```python
from build123d import *

# Parameters (mm, degrees)
F1_DEPTH = 5.2
F3_DEPTH = 25.4


with BuildPart() as f1:
    # F0 (on Front) → F1 (new body)
    with BuildSketch(Plane.XZ):
        Polygon((1.5, 0), (0, 0), (0, -12), (12, -12), (12, -10.8), (1.5, -10.8), align=None)
    extrude(amount=-F1_DEPTH)

    # F2 (on face) → F3 (cut)
    with BuildSketch(Plane.YZ.offset(1.5)):
        with BuildLine():
            Line((1.1, -2.9), (1.1, -7.9))
            ThreePointArc((1.1, -7.9), (2.575413, -9.400208), (4.1, -7.95))
            Line((4.1, -7.95), (4.1, -2.9))
            ThreePointArc((4.1, -2.9), (2.6, -1.4), (1.1, -2.9))
        make_face()
    extrude(amount=-F3_DEPTH, mode=Mode.SUBTRACT)


solid = f1.part
```
Check sheet for the modelled part. Datum: model origin and axes. Units: mm. A direction names the side the tool comes from. Round coordinates to 2 decimals unless told otherwise and drop trailing zeros. Order: outer loops, then holes, each group sorted by start corner. A loop starts at its lowest first (then second) coordinate and runs counter-clockwise, first axis right, second up. Notation, with made-up numbers: (16, 81) -> (59, 81) arc R26 ccw to (59, 114) -> close; hole circle Ø4 at (-30, 63). An arc over 180 degrees is marked (long way). One line per item, written item: value. Start each with the question number.
Q1. Cross-section at C-C (y = 4.7). Record the boundary of the cut face in (x, z).
Q2. Cross-section at D-D (y = 3.35). Record the boundary of the cut face in (x, z).
Q3. Mould release check, pull along Z, two halves, no side actions. Record for faces 1 (the face through (3, 5.2, -11)), 2 (the face through (1, 1.1, -5)), 3 (the face through (1, 3, 0)): pulls with the +Z half, pulls with the -Z half, needs draft (parallel to the pull), parting line crosses it, or undercut.
Q4. Cross-section at A-A (z = -3.5). Record the boundary of the cut face in (x, y).
Q5. Gauge pin test, flat ends, axial feed: pin 1 Ø1.5 at (x, z) = (4, -4) entering from +Y; pin 2 Ø1.2 at (x, z) = (1, -5.5) entering from -Y. Record the tip position at first contact, or that the pin passes through.
Q6. Cross-section at B-B (y = 2.6). Record the boundary of the cut face in (x, z), and give its area (3 significant figures).
Q7. Thickness scan on line 1 (Y direction, x = 0.5, z = -4); line 2 (Z direction, x = 11, y = 4.55); line 3 (X direction, y = 5, z = -9.5). Record the ranges inside material, lowest first.
Q8. Set-up check for faces 4 (the face through (7, 3, -10.8)), 5 (the face through (0.76, 2.54, -9.4)), 6 (the face through (3, 0, -11)): record each of +Z, -Z, +X, -X, +Y, -Y from which the full face is reachable in a straight line by a thin tool's end or side.
Completed:
1. outline: (0, -12) -> (12, -12) -> (12, -10.8) -> (1.5, -10.8) -> (1.5, 0) -> (0, 0) -> close
2. outline: (0, -12) -> (12, -12) -> (12, -10.8) -> (1.5, -10.8) -> (1.5, -9.2) -> (0, -9.2) -> close; (0, -1.6) -> (1.5, -1.6) -> (1.5, 0) -> (0, 0) -> close
3. face 1: needs draft
3. face 2: undercut
3. face 3: pulls with the +Z half
4. outline: (0, 0) -> (1.5, 0) -> (1.5, 1.1) -> (0, 1.1) -> close; (0, 4.1) -> (1.5, 4.1) -> (1.5, 5.2) -> (0, 5.2) -> close
5. pin 1: passes through
5. pin 2: stops at y = 0
6. outline: (0, -12) -> (12, -12) -> (12, -10.8) -> (1.5, -10.8) -> (1.5, -9.4) -> (0, -9.4) -> close; (0, -1.4) -> (1.5, -1.4) -> (1.5, 0) -> (0, 0) -> close
6. area: 18.6 mm²
7. line 1: y = 0 to 1.1, 4.1 to 5.2
7. line 2: z = -12 to -10.8
7. line 3: x = 0 to 1.5
8. face 4: +Z, +X, +Y, -Y
8. face 5: +X, -X
8. face 6: +Z, -Z, +X, -X, -Y
